Autodesk Inventor part; units mm, degrees
ref_plane "YZ Plane" through (0, 0, 0) normal (1, 0, 0) x (0, 1, 0)
ref_plane "XZ Plane" through (0, 0, 0) normal (0, 1, 0) x (-1, 0, 0)
ref_plane "XY Plane" through (0, 0, 0) normal (0, 0, 1) x (1, 0, 0)
sketch "Sketch1" plane through (0, 0, 0) normal (0, 1, 0) x (-1, 0, 0)
  circle A0 centre (0, 0) radius 18.3769
  line L0 (18.3769, 18.3769) -> (-18.3769, -18.3769) construction
  line L1 (-18.3769, 18.3769) -> (18.3769, -18.3769) construction
  line L2 (13.335, 21.59) -> (-13.335, 21.59)
  line L3 (-21.59, 13.335) -> (-21.59, -13.335)
  line L4 (-13.335, -21.59) -> (13.335, -21.59)
  line L5 (21.59, -13.335) -> (21.59, 13.335)
  line L6 (21.59, 21.59) -> (-21.59, -21.59) construction
  line L7 (-21.59, 21.59) -> (21.59, -21.59) construction
  line L8 (21.59, 13.335) -> (13.335, 21.59)
  line L9 (-13.335, 21.59) -> (-21.59, 13.335)
  line L10 (-21.59, -13.335) -> (-13.335, -21.59)
  line L11 (13.335, -21.59) -> (21.59, -13.335)
  circle A1 centre (15.24, -15.24) radius 1.0033
  circle A2 centre (-15.24, -15.24) radius 1.0033
  circle A3 centre (-15.24, 15.24) radius 1.0033
  circle A4 centre (15.24, 15.24) radius 1.0033
  line L12 (11.9917, -21.9869) -> (-11.9917, -21.9869)
  line L13 (-21.9869, -11.9917) -> (-21.9869, 11.9917)
  line L14 (-11.9917, 21.9869) -> (11.9917, 21.9869)
  line L15 (21.9869, 11.9917) -> (21.9869, -11.9917)
  line L16 (-20.3962, 23.5712) -> (20.3962, 23.5712)
  line L17 (23.5712, 20.3962) -> (23.5712, -20.3962)
  line L18 (20.3962, -23.5712) -> (-20.3962, -23.5712)
  line L19 (-23.5712, -20.3962) -> (-23.5712, 20.3962)
  line L20 (-23.5712, 23.5712) -> (23.5712, -23.5712) construction
  line L21 (23.5712, 23.5712) -> (-23.5712, -23.5712) construction
  arc A5 (20.3962, -23.5712) -> (23.5712, -20.3962) centre (20.3962, -20.3962) ccw
  arc A6 (-23.5712, -20.3962) -> (-20.3962, -23.5712) centre (-20.3962, -20.3962) ccw
  arc A7 (-20.3962, 23.5712) -> (-23.5712, 20.3962) centre (-20.3962, 20.3962) ccw
  arc A8 (23.5712, 20.3962) -> (20.3962, 23.5712) centre (20.3962, 20.3962) ccw
  circle A9 centre (20.3962, -20.3962) radius 1.0033
  circle A10 centre (-20.3962, -20.3962) radius 1.0033
  circle A11 centre (-20.3962, 20.3962) radius 1.0033
  circle A12 centre (20.3962, 20.3962) radius 1.0033
  line L22 (16.4818, -20.127) -> (20.127, -16.4818)
  line L23 (20.127, 16.4818) -> (16.4818, 20.127)
  line L24 (-16.4818, 20.127) -> (-20.127, 16.4818)
  line L25 (-20.127, -16.4818) -> (-16.4818, -20.127)
  arc A13 (21.9869, 11.9917) -> (20.127, 16.4818) centre (15.6369, 11.9917) ccw
  arc A14 (16.4818, 20.127) -> (11.9917, 21.9869) centre (11.9917, 15.6369) ccw
  arc A15 (-11.9917, 21.9869) -> (-16.4818, 20.127) centre (-11.9917, 15.6369) ccw
  arc A16 (-20.127, 16.4818) -> (-21.9869, 11.9917) centre (-15.6369, 11.9917) ccw
  arc A17 (-21.9869, -11.9917) -> (-20.127, -16.4818) centre (-15.6369, -11.9917) ccw
  arc A18 (-16.4818, -20.127) -> (-11.9917, -21.9869) centre (-11.9917, -15.6369) ccw
  arc A19 (11.9917, -21.9869) -> (16.4818, -20.127) centre (11.9917, -15.6369) ccw
  arc A20 (20.127, -16.4818) -> (21.9869, -11.9917) centre (15.6369, -11.9917) ccw
  line L26 (4.3815, -5.969) -> (4.3815, -12.5476)
  line L27 (2.794, -14.1351) -> (-2.794, -14.1351)
  line L28 (-4.3815, -12.5476) -> (-4.3815, -5.969)
  line L29 (4.3815, 5.969) -> (4.3815, 12.5476)
  line L30 (2.794, 14.1351) -> (-2.794, 14.1351)
  line L31 (-4.3815, 12.5476) -> (-4.3815, 5.969)
  line L32 (-5.969, -4.3815) -> (-12.5476, -4.3815)
  line L33 (-14.1351, -2.794) -> (-14.1351, 2.794)
  line L34 (-12.5476, 4.3815) -> (-5.969, 4.3815)
  line L35 (5.969, -4.3815) -> (12.5476, -4.3815)
  line L36 (14.1351, -2.794) -> (14.1351, 2.794)
  line L37 (12.5476, 4.3815) -> (5.969, 4.3815)
  arc A21 (2.794, -14.1351) -> (4.3815, -12.5476) centre (2.794, -12.5476) ccw
  arc A22 (-4.3815, -12.5476) -> (-2.794, -14.1351) centre (-2.794, -12.5476) ccw
  arc A23 (-4.3815, -5.969) -> (-5.969, -4.3815) centre (-5.969, -5.969) ccw
  arc A24 (-14.1351, -2.794) -> (-12.5476, -4.3815) centre (-12.5476, -2.794) ccw
  arc A25 (-14.1351, -2.794) -> (-12.5476, -4.3815) centre (-12.5476, -2.794) ccw
  arc A26 (-12.5476, 4.3815) -> (-14.1351, 2.794) centre (-12.5476, 2.794) ccw
  arc A27 (-5.969, 4.3815) -> (-4.3815, 5.969) centre (-5.969, 5.969) ccw
  arc A28 (-2.794, 14.1351) -> (-4.3815, 12.5476) centre (-2.794, 12.5476) ccw
  arc A29 (4.3815, 12.5476) -> (2.794, 14.1351) centre (2.794, 12.5476) ccw
  arc A30 (4.3815, 5.969) -> (5.969, 4.3815) centre (5.969, 5.969) ccw
  arc A31 (14.1351, 2.794) -> (12.5476, 4.3815) centre (12.5476, 2.794) ccw
  arc A32 (12.5476, -4.3815) -> (14.1351, -2.794) centre (12.5476, -2.794) ccw
  arc A33 (5.969, -4.3815) -> (4.3815, -5.969) centre (5.969, -5.969) ccw
  line L38 (-2.794, -14.9289) -> (2.794, -14.9289)
  arc A34 (2.794, -14.9289) -> (5.1753, -12.5476) centre (2.794, -12.5476) ccw
  line L39 (5.1753, -12.5476) -> (5.1753, -5.969)
  arc A35 (5.969, -5.1753) -> (5.1753, -5.969) centre (5.969, -5.969) ccw
  line L40 (5.969, -5.1753) -> (12.5476, -5.1753)
  arc A36 (12.5476, -5.1753) -> (14.9289, -2.794) centre (12.5476, -2.794) ccw
  line L41 (14.9289, -2.794) -> (14.9289, 2.794)
  arc A37 (14.9289, 2.794) -> (12.5476, 5.1753) centre (12.5476, 2.794) ccw
  line L42 (12.5476, 5.1753) -> (5.969, 5.1753)
  arc A38 (5.1753, 5.969) -> (5.969, 5.1753) centre (5.969, 5.969) ccw
  line L43 (5.1753, 5.969) -> (5.1753, 12.5476)
  arc A39 (5.1753, 12.5476) -> (2.794, 14.9289) centre (2.794, 12.5476) ccw
  line L44 (2.794, 14.9289) -> (-2.794, 14.9289)
  arc A40 (-2.794, 14.9289) -> (-5.1753, 12.5476) centre (-2.794, 12.5476) ccw
  line L45 (-5.1753, 12.5476) -> (-5.1753, 5.969)
  arc A41 (-5.969, 5.1753) -> (-5.1753, 5.969) centre (-5.969, 5.969) ccw
  line L46 (-5.969, 5.1753) -> (-12.5476, 5.1753)
  arc A42 (-12.5476, 5.1753) -> (-14.9289, 2.794) centre (-12.5476, 2.794) ccw
  line L47 (-14.9289, 2.794) -> (-14.9289, -2.794)
  arc A43 (-14.9289, -2.794) -> (-12.5476, -5.1753) centre (-12.5476, -2.794) ccw
  line L48 (-12.5476, -5.1753) -> (-5.969, -5.1753)
  arc A44 (-5.1753, -5.969) -> (-5.969, -5.1753) centre (-5.969, -5.969) ccw
  line L49 (-5.1753, -5.969) -> (-5.1753, -12.5476)
  arc A45 (-5.1753, -12.5476) -> (-2.794, -14.9289) centre (-2.794, -12.5476) ccw
  line L50 (11.9917, -21.59) -> (-11.9917, -21.59)
  line L51 (-11.9917, -21.59) -> (-11.9917, -13.9252)
  line L52 (11.9917, -13.9252) -> (11.9917, -21.59)
  point P0 (4.3815, -14.1351)
  point P1 (-4.3815, -14.1351)
  point P2 (4.3815, 14.1351)
  point P3 (-14.1351, 4.3815)
  point P4 (-4.3815, 4.3815)
  point P5 (14.1351, 4.3815)
  point P6 (4.3815, 4.3815)
  dimension "d33" = 36.7538
  dimension "d34" = 43.18
  dimension "d35" = 43.18
  dimension "d48" = 2.0066
  dimension "d49" = 2.0066
  dimension "d50" = 2.0066
  dimension "d51" = 2.0066
  dimension "d52" = 0.3969
  dimension "d53" = 47.1424
  dimension "d54" = 47.1424
  dimension "d55" = 3.175
  dimension "d56" = 2.0066
  dimension "d57" = 2.0066
  dimension "d58" = 2.0066
  dimension "d59" = 2.0066
  dimension "d62" = 6.35
  dimension "d79" = 8.763
  dimension "d84" = 1.5875
  dimension "d85" = 0.7937
  dimension "d86" = 9.7536
extrude "outer" add sketch "Sketch1" along normal blind 12.7 contours L16 A8 L17 A5 L18 A6 L19 A7
extrude "pcb support" add sketch "Sketch1" along normal blind 9.525 contours A0 L51 L4 L10 L3 L9 L2 L8 L5 L11 L52 | A0 L52 L4 L51 | L12 A18 L25 A17 L13 A16 L24 A15 L14 A14 L23 A13 L15 A20 L22 A19
extrude "pcb screw hole location" add sketch "Sketch1" along normal blind 9.525 contours A1 | A2 | A3 | A4
extrude "back cover screw hole location" add sketch "Sketch1" along normal blind 12.7 contours A9 | A10 | A11 | A12
extrude "dpad face" add sketch "Sketch1" along normal blind 1.5875 contours A0
sketch "Sketch3" plane through (20.3962, 0, -23.5712) normal (0, 0, -1) x (-1, 0, 0)
  line L0 (0, 0) -> (40.7924, 0)
  line L1 (-3.175, 0) -> (-3.175, 12.7)
  line L2 (32.3879, 9.525) -> (8.4045, 9.525)
  line L3 (8.4045, 9.525) -> (32.3879, 9.525)
  circle A0 centre (20.3962, 9.525) radius 3.9687
  point P0 (20.3962, 0)
  dimension "d92" = 7.9375
extrude "ether cable" [suppressed]
sketch "Sketch4" plane through (0, 9.525, 0) normal (0, 1, 0) x (1, 0, 0)
  circle A0 centre (0, 0) radius 18.3769
  line L0 (11.9917, 21.9869) -> (-11.9917, 21.9869)
  line L1 (-11.9917, 21.9869) -> (11.9917, 21.9869)
  line L2 (11.9917, 21.9869) -> (11.9917, 13.9252)
  line L3 (-11.9917, 13.9252) -> (-11.9917, 21.9869)
  arc A1 (11.9917, 13.9252) -> (-11.9917, 13.9252) centre (0, 0) ccw
extrude "pocket" cut sketch "Sketch4" against normal blind 1.5875 contours A0 L3 L0 L2
properties part number "SnakeControllerCase_v3"
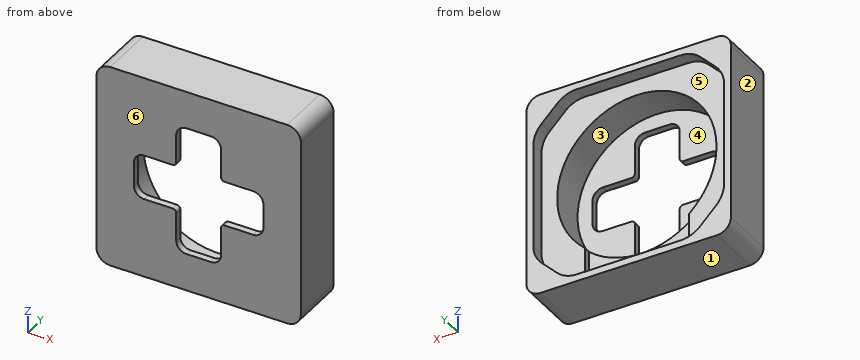
Geometry check sheet. Reference: the model listing, model coordinates, mm. Face numbers are marked on the shaded views. A direction names the side the tool comes from. Round coordinates to 2 decimals unless told otherwise and drop trailing zeros. Loops run counter-clockwise (first coordinate to the right, second up) from the corner with the lowest first, then second, coordinate; pieces in that order, holes last. Notation, with made-up numbers: (16.25, 82.5) -> (71.25, 82.5) arc R30 cw to (71.25, 115.5) -> close; hole circle Ø6 at (76.5, 67). An arc over 180 degrees is marked (long way). Use a Markdown table: item, result.
(1) Sectioned sample at B-B (x = 14). Enter the section's corners in (y, z) (1 decimal).
Calculated:
| item | result |
|---|---|
| outline | (0, -23.6) -> (12.7, -23.6) -> (12.7, -21.7) -> (9.5, -21.7) -> (9.5, -11.9) -> (1.6, -11.9) -> (1.6, -4.7) -> (0, -4.7) -> close; (0, 4.7) -> (1.6, 4.7) -> (1.6, 11.9) -> (9.5, 11.9) -> (9.5, 21.7) -> (12.7, 21.7) -> (12.7, 23.6) -> (0, 23.6) -> close |
(2) Sectioned sample at C-C (y = 6.5). Enter the section's corners in (x, z) (3 decimals), then the cut area to 3 significant figures.
Calculated:
| item | result |
|---|---|
| outline | (-23.571, -20.396) arc R3.175 ccw to (-20.396, -23.571) -> (20.396, -23.571) arc R3.175 ccw to (23.571, -20.396) -> (23.571, 20.396) arc R3.175 ccw to (20.396, 23.571) -> (-20.396, 23.571) arc R3.175 ccw to (-23.571, 20.396) -> close; hole circle Ø36.754 at (0, 0) |
| area | 1,150 mm² |
(3) Set-up check for the marked faces 5 and 6: record each of +Z, -Z, +X, -X, +Y, -Y from which the full face is reachable in a straight line by a thin tool's end or side.
Calculated:
| item | result |
|---|---|
| face 5 | +Y |
| face 6 | +Z, -Z, +X, -X, -Y |
(4) Sectioned sample at D-D (z = -19). Enter the section's corners in (x, y) (1 decimal).
Calculated:
| item | result |
|---|---|
| outline | (-23.6, 0) -> (23.6, 0) -> (23.6, 12.7) -> (17.6, 12.7) -> (17.6, 9.5) -> (12, 9.5) -> (12, 7.9) -> (-12, 7.9) -> (-12, 9.5) -> (-17.6, 9.5) -> (-17.6, 12.7) -> (-23.6, 12.7) -> close |
(5) Mould release check, pull along Z, two halves, no side actions. Record for the marked faces 1, 2, 3 and 4: released by +Z, released by -Z, zero draft, split by the parting line, or undercut.
Calculated:
| item | result |
|---|---|
| face 1 | released by -Z |
| face 2 | zero draft |
| face 3 | undercut |
| face 4 | undercut |
(6) Sectioned sample at A-A (z = 0). Enter the section's corners in (x, y) (1 decimal).
Calculated:
| item | result |
|---|---|
| outline | (-23.6, 0) -> (-14.9, 0) -> (-14.9, 1.6) -> (-18.4, 1.6) -> (-18.4, 9.5) -> (-22, 9.5) -> (-22, 12.7) -> (-23.6, 12.7) -> close; (14.9, 0) -> (23.6, 0) -> (23.6, 12.7) -> (22, 12.7) -> (22, 9.5) -> (18.4, 9.5) -> (18.4, 1.6) -> (14.9, 1.6) -> close |
(7) Go/stop test with flat-tipped pins: P1, Ø2, axis at x = -7, z = -12.5, coming from the +Y side; P2, Ø1, axis at x = 12, z = -18.5, coming from the +Y side (3 decimals); P3, Ø10, axis at x = 7.5, z = -7.5, coming from the -Y side. Record where each tip stops, or that it passes through.
Calculated:
| item | result |
|---|---|
| P1 | y = 1.59 |
| P2 | y = 9.525 |
| P3 | y = 0 |
(8) Scan lines: probe 1 along Z at (x, y) = (0, 3.25); probe 2 along Z at (x, y) = (0.5, 8.75). Record each from-to range of solid material in increasing order.
Calculated:
| item | result |
|---|---|
| probe 1 | -23.57 to -18.38, 18.38 to 23.57 |
| probe 2 | -23.57 to -21.99, 18.37 to 23.57 |
